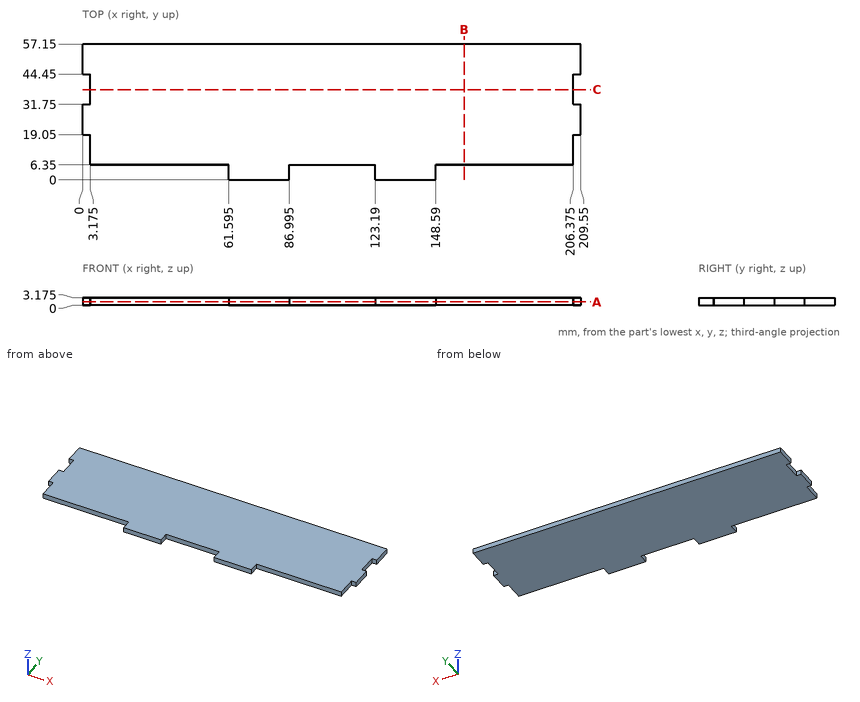
Print and shaded views of the part. All mm, measured from the part's lowest x, y and z. Round coordinates to 2 decimals unless told otherwise and drop trailing zeros. Write each loop counter-clockwise with the first axis right and the second up, starting at its lowest first coordinate (ties: lowest second). Pieces come first, ordered by that corner, then holes. Notation, with made-up numbers: M -1,76.25 L 24,76.25 A12 cw 24,95.25 Z; hole C 50.25,-7 d2. An arc over 180 degrees is marked long. One line per question, with ' | ' between items.
(1) Saw through at B-B on x = 160.5. Write the cut outline in (y, z) (3 decimals).
Answer key:
outline: M 6.35,0 L 57.15,0 L 57.15,3.175 L 6.35,3.175 Z
(2) Pin check, flat tips, straight feed: pin 1 (3 mm diameter, centred on x = 51, y = 12, fed in from -Z); pin 2 (1.6 mm diameter, centred on x = 106, z = 2, fed in from -Y); pin 3 (1 mm diameter, centred on y = 37, z = 1, fed in from +X) (3 decimals); pin 4 (1.6 mm diameter, centred on y = 11, z = 1, fed in from -X) (3 decimals). Stop position of each tip, or through.
Answer key:
pin 1: stops at z = 0 | pin 2: stops at y = 6.35 | pin 3: stops at x = 206.375 | pin 4: stops at x = 3.175
(3) Saw through at C-C on y = 38. Write the cut outline in (x, z) (3 decimals), then the cut area to 3 significant figures.
Answer key:
outline: M 3.175,0 L 206.375,0 L 206.375,3.175 L 3.175,3.175 Z | area: 645 mm^2
(4) Saw through at A-A on z = 1.5. Write the cut outline in (x, y) (3 decimals), then the cut area to 3 significant figures.
Answer key:
outline: M 0,19.05 L 3.175,19.05 L 3.175,6.35 L 61.595,6.35 L 61.595,0 L 86.995,0 L 86.995,6.35 L 123.19,6.35 L 123.19,0 L 148.59,0 L 148.59,6.35 L 206.375,6.35 L 206.375,19.05 L 209.55,19.05 L 209.55,31.75 L 206.375,31.75 L 206.375,44.45 L 209.55,44.45 L 209.55,57.15 L 0,57.15 L 0,44.45 L 3.175,44.45 L 3.175,31.75 L 0,31.75 Z | area: 10,800 mm^2
(5) Probe line 1 along X through (y, z) = (3, 2.65) (3 decimals); line 2 along Y through (x, z) = (43, 2.2); line 3 along X through (y, z) = (16, 1.7) (3 decimals). List the from-to ranges inside material, lowest first.
Answer key:
line 1: x = 61.595 to 86.995, 123.19 to 148.59 | line 2: y = 6.35 to 57.15 | line 3: x = 3.175 to 206.375
